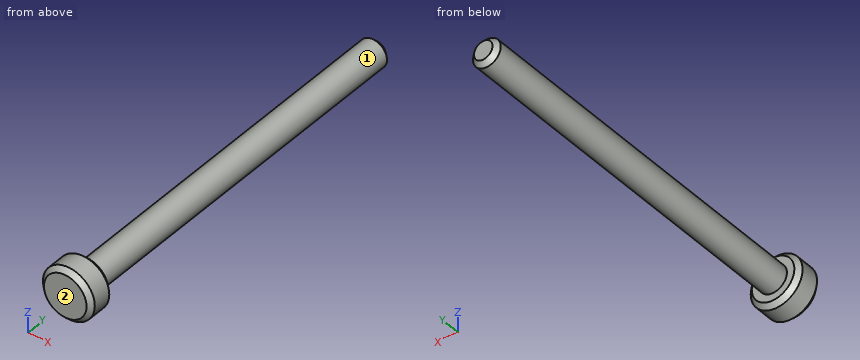
```python
from build123d import *

# Parameters (mm, degrees)
SKETCH1_R           = 2.8
BOSS_EXTRUDE1_DEPTH = 1.5
SKETCH2_R           = 1.5
BOSS_EXTRUDE2_DEPTH = 40
CHAMFER1_SIZE       = 0.5
CHAMFER2_SIZE       = 0.5


with BuildPart() as part:
    # Sketch1 → Boss-Extrude1 (new body, symmetric)
    with BuildSketch(Plane(origin=(0, 0, 0), x_dir=(1, 0, 0), z_dir=(0, 1, 0))):
        Circle(SKETCH1_R)
    extrude(amount=BOSS_EXTRUDE1_DEPTH, both=True)

    # Sketch2 → Boss-Extrude2 (add)
    with BuildSketch(Plane(origin=(0, 1.5, 0), x_dir=(1, 0, 0), z_dir=(0, 1, 0))):
        Circle(SKETCH2_R)
    extrude(amount=BOSS_EXTRUDE2_DEPTH)

    # Chamfer1
    chamfer1_edges = [part.edges().sort_by_distance(p)[0] for p in [
        (-1.5, 41.5, 0),
    ]]
    chamfer(chamfer1_edges, length=CHAMFER1_SIZE)

    # Chamfer2
    chamfer2_edges = [part.edges().sort_by_distance(p)[0] for p in [
        (-2.8, -1.5, 0),
        (-2.8, 1.5, 0),
    ]]
    chamfer(chamfer2_edges, length=CHAMFER2_SIZE)


solid = part.part
```
Check sheet for the modelled part. Datum: model origin and axes. Units: mm. Face numbers are marked on the shaded views. A direction names the side the tool comes from. Give positions to 0.01 mm unless a question says otherwise; leave off trailing zeros. Write each loop counter-clockwise with the first axis right and the second up, starting at its lowest first coordinate (ties: lowest second). Pieces come first, ordered by that corner, then holes. Notation, with made-up numbers: (-9, -16.75) - (20, -16.75) arc R22 ccw to (20, -4.75) - close; hole circle Ø8 at (70, -7.5). An arc over 180 degrees is marked (long way). Answer as a JSON object with one key per item and string values. Group by question number.
1) Sectioned sample at A-A (x = 0). Record the cut outline in (y, z), then the cut area to 3 significant figures.
2) Sectioned sample at B-B (z = 0). Record the cut outline in (x, y), then the cut area to 3 significant figures.
3) Sectioned sample at C-C (y = 9.5). Record the cut outline in (x, z), then the cut area to 3 significant figures.
4) Thickness scan on probe 1 along Y at (x, z) = (0.1, -2); probe 2 along Z at (x, y) = (-0.15, 10); probe 3 along X at (y, z) = (6, -0.85). Record the ranges inside material, lowest first. Write a range as from..to.
5) Access from +Z, -Z, +X, -X, +Y, -Y to the whole of each face (thin tool, end or side, straight path). Record for the marked faces 1 and 2.
6) Depth check by flat-ended pin: P1, Ø1.5, axis at y = 28.5, z = -2, coming from the -X side; P2, Ø2, axis at x = -2, z = 1, coming from the +Y side; P3, Ø3, axis at y = 30, z = -1.5, coming from the +X side. Enter the tip coordinate at first touch or a pass-through.
Geometry results:
{
 "1": {"outline": "(-1.5, -2.3) - (-1, -2.8) - (1, -2.8) - (1.5, -2.3) - (1.5, -1.5) - (41, -1.5) - (41.5, -1) - (41.5, 1) - (41, 1.5) - (1.5, 1.5) - (1.5, 2.3) - (1, 2.8) - (-1, 2.8) - (-1.5, 2.3) - close", "area": "136 mm^2"},
 "2": {"outline": "(-2.8, -1) - (-2.3, -1.5) - (2.3, -1.5) - (2.8, -1) - (2.8, 1) - (2.3, 1.5) - (1.5, 1.5) - (1.5, 41) - (1, 41.5) - (-1, 41.5) - (-1.5, 41) - (-1.5, 1.5) - (-2.3, 1.5) - (-2.8, 1) - close", "area": "136 mm^2"},
 "3": {"outline": "circle Ø3 at (0, 0)", "area": "7.07 mm^2"},
 "4": {"probe 1": "y = -1.5..1.5", "probe 2": "z = -1.49..1.49", "probe 3": "x = -1.24..1.24"},
 "5": {"face 1": "+Y", "face 2": "+Z, -Z, +X, -X, -Y"},
 "6": {"P1": "stops at x = -0.83", "P2": "stops at y = 41.26", "P3": "stops at x = 1.5"}
}
